Geometry: final body of the model. Coordinates: model frame, mm. A direction names the side the tool comes from. Give positions to 0.01 mm unless a question says otherwise; leave off trailing zeros. Write each loop counter-clockwise with the first axis right and the second up, starting at its lowest first coordinate (ties: lowest second). Pieces come first, ordered by that corner, then holes. Notation, with made-up numbers: (60.5, 43.5) -> (95.5, 43.5) arc R34 ccw to (95.5, 80.5) -> close; hole circle Ø2 at (20.25, 54). An arc over 180 degrees is marked (long way). Answer in a Markdown table with one row per item. Add a question column.
Item 1: Draft query along X for faces 1 (the cylindrical face through (-36.534, -15.697, -28.013)), 2 (the cylindrical face through (-0.86, -15.653, -3.874)), 3 (the flat face through (5, -31.75, 0)). Return one class per face: +X half, -X half, draft (parallel to the pull), parting line (faces both ways), or undercut.
Item 2: Access query for faces 4 (the cylindrical face through (-5.506, -30.185, -24.796)), 5 (the flat face through (5, 0, 0)), 6 (the flat face through (-20, -3.175, -20)). Directions: +Z, -Z, +X, -X, +Y, -Y. A direction counts if a zero-diameter tool reaches every point of the face in a straight line with its end or side. Return the directions, or none.
Item 3: Section query D-D on y = -11. Output: boundary loops of the cut face in (x, z) (1 decimal).
Item 4: First-contact query: P1, Ø12, axis at y = -11.5, z = 25, coming from the +X side; P2, Ø2, axis at x = -7.5, y = -19, coming from the +Z side; P3, Ø3, axis at x = -35.5, y = -21.5, coming from the -Z side; P4, Ø7, axis at x = 0, z = 0, coming from the +Y side. Flat tips, straight axial feed; report the tip coordinate or a pass-through.
Item 5: Material intervals for probe 1 along Z at (x, y) = (0, -7); probe 2 along Y at (x, z) = (7, -37.5) (3 decimals); probe 3 along X at (y, z) = (-14.5, 2), sorted ascending. Write a range as from..to.
Item 6: Section query C-C on z = 22.5. Output: boundary loops of the cut face in (x, y) (3 decimals).
```python
from build123d import *

# Parameters (mm, degrees)
F0_R     = 46.0375
F1_DEPTH = 31.75
F2_R     = 46.0375
F2_R_2   = 25.4
F3_DEPTH = 3.175
F4_R     = 46.0375
F4_R_2   = 25.4
F5_DEPTH = 3.175
F6_R     = 3.96875
F7_DEPTH = 31.751


with BuildPart() as f1:
    # F0 (on Front) → F1 (new body)
    with BuildSketch(Plane.XZ):
        Circle(F0_R)
    extrude(amount=F1_DEPTH)

    # F2 (on face) → F3 (cut)
    with BuildSketch(Plane.XZ.offset(31.75)):
        Circle(F2_R)
        Circle(F2_R_2, mode=Mode.SUBTRACT)
    extrude(amount=-F3_DEPTH, mode=Mode.SUBTRACT)

    # F4 (on face) → F5 (cut)
    with BuildSketch(Plane(origin=(0, 0, 0), x_dir=(-1, 0, 0), z_dir=(0, 1, 0))):
        Circle(F4_R)
        Circle(F4_R_2, mode=Mode.SUBTRACT)
    extrude(amount=-F5_DEPTH, mode=Mode.SUBTRACT)

    # F6 (on Front) → F7 (cut, through all)
    with BuildSketch(Plane.XZ):
        Circle(F6_R)
    extrude(amount=F7_DEPTH, mode=Mode.SUBTRACT)


solid = f1.part
```
Findings below:
| question | item | result |
|---|---|---|
| 1 | face 1 | parting line |
| 1 | face 2 | undercut |
| 1 | face 3 | draft |
| 2 | face 4 | -Y |
| 2 | face 5 | +Z, -Z, +X, -X, +Y |
| 2 | face 6 | +Y |
| 3 | outline | circle Ø92.1 at (0, 0); hole circle Ø7.9 at (0, 0) |
| 4 | P1 | stops at x = 41.93 |
| 4 | P2 | stops at z = 45.58 |
| 4 | P3 | stops at z = -31.04 |
| 4 | P4 | passes through |
| 5 | probe 1 | z = -46.04..-3.97, 3.97..46.04 |
| 5 | probe 2 | y = -28.575..-3.175 |
| 5 | probe 3 | x = -45.99..-3.43, 3.43..45.99 |
| 6 | outline | (-40.165, -28.575) -> (-11.786, -28.575) -> (-11.786, -31.75) -> (11.786, -31.75) -> (11.786, -28.575) -> (40.165, -28.575) -> (40.165, -3.175) -> (11.786, -3.175) -> (11.786, 0) -> (-11.786, 0) -> (-11.786, -3.175) -> (-40.165, -3.175) -> close |
